Geometry: final body of the model. Coordinates: model frame, mm. Give positions to 0.01 mm unless a question says otherwise; leave off trailing zeros. Loops run counter-clockwise (first coordinate to the right, second up) from the corner with the lowest first, then second, coordinate; pieces in that order, holes last. Notation, with made-up numbers: (28, 35.5) - (57, 35.5) arc R17 cw to (57, 48.5) - close; hole circle Ø5 at (59, 62). An arc over 180 degrees is marked (long way). Use one line per item in the form item = value.
```python
from build123d import *

# Parameters (mm, degrees)
EXTRUDE_1_DEPTH     = 3.2
SKETCH_5_R          = 2.5
CUT_EXTRUDE_1_DEPTH = 7.897342483
CHAMFER_1_SIZE      = 0.2


with BuildPart() as part:
    # Эскиз1 → Вытянуть1 (new body)
    with BuildSketch(Plane(origin=(0, 0, 0), x_dir=(1, 0, 0), z_dir=(0, 1, 0))):
        Polygon((-2.309401077, 4), (2.309401077, 4), (4.618802154, 0), (2.309401077, -4), (-2.309401077, -4), (-4.618802154, 0), align=None)
    extrude(amount=-EXTRUDE_1_DEPTH)

    # Эскиз5 → Вырез-Вытянуть1 (cut, through all)
    with BuildSketch(Plane.XZ.offset(3.2)):
        with Locations(Location((0, 0, 0), (0, 0, 270))):
            Circle(SKETCH_5_R)
    extrude(amount=-CUT_EXTRUDE_1_DEPTH, mode=Mode.SUBTRACT)

    # Эскиз4 → Вырез-Повернуть1 (revolve, cut)
    with BuildSketch(Plane.XY):
        Polygon((-4.618802154, -0.5), (-4.118802154, 0), (-4.618802154, 0), align=None)
        Polygon((-4.618802154, -2.7), (-4.118802154, -3.2), (-4.618802154, -3.2), align=None)
    revolve(axis=Axis((0, 0, 0), (0, -1, 0)), mode=Mode.SUBTRACT)

    # Фаска1
    chamfer_1_edges = [part.edges().sort_by_distance(p)[0] for p in [
        (0, 0, 2.5),
        (0, -3.2, 2.5),
    ]]
    chamfer(chamfer_1_edges, length=CHAMFER_1_SIZE)


solid = part.part
```
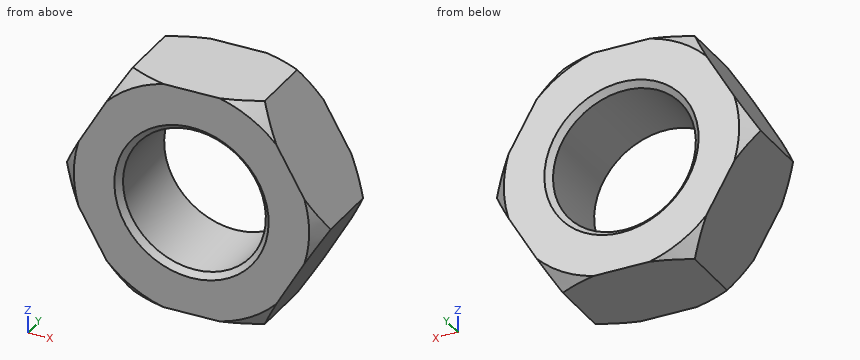
(1) Material intervals for L1, parallel to X at y = -2.1, z = 0.5; L2, parallel to Z at x = 2, y = -0.15; L3, parallel to Z at x = -1.5, y = -2.85, sorted ascending. Write a range as from..to.
Solution:
L1 = -4.33..-2.45, 2.45..4.33
L2 = -3.77..-1.58, 1.58..3.77
L3 = -4..-2, 2..4
(2) Pin query (flat end, axial travel): P1, Ø1.5, axis at y = -0.5, z = -3, coming from the -X side. Return the tip coordinate at first contact, or that it passes through.
Solution:
P1 = -3.32
(3) Cut plane A-A (y = -0.8). Return the cut outline in (x, z), plus the area to 3 significant figures.
Solution:
outline = (-4.62, 0) - (-2.31, -4) - (2.31, -4) - (4.62, 0) - (2.31, 4) - (-2.31, 4) - close; hole circle Ø5 at (0, 0)
area = 35.8 mm2
(4) Cut plane B-B (x = -3.5). Return the cut outline in (y, z), plus the area to 3 significant figures.
Solution:
outline = (-3.2, -1.94) - (0, -1.94) - (0, 1.94) - (-3.2, 1.94) - close
area = 12.4 mm2
